Autodesk Inventor part; units mm, degrees
ref_plane "Work Plane1" through (0, 0, -6.2) normal (0, 0, -1) x (-1, 0, 0)
ref_plane "YZ Plane" through (0, 0, 0) normal (1, 0, 0) x (0, 1, 0)
ref_plane "XZ Plane" through (0, 0, 0) normal (0, 1, 0) x (-1, 0, 0)
sketch "Sketch1" plane through (0, 0, 0) normal (0, 0, 1) x (1, 0, 0)
  circle A0 centre (0, 0) radius 9.375
  dimension "d0" = 18.75
extrude "Extrusion1" add sketch "Sketch1" along normal blind 32
sketch "Sketch2" plane through (0, 0, 32) normal (0, 0, 1) x (1, 0, 0)
  circle A0 centre (0, 0) radius 9.375
  circle A1 centre (0, 0) radius 6.8
  dimension "d3" = 13.6
extrude "Extrusion2" add sketch "Sketch2" along normal blind 3.3 contours A1
sketch "Sketch3" plane through (0, 0, 32) normal (0, 0, 1) x (1, 0, 0)
  circle A0 centre (0, 0) radius 6.8
  line L0 (-3.25, 8) -> (3.25, 8)
  line L1 (-3.25, -8) -> (3.25, -8)
  line L2 (-3.25, 8) -> (-3.25, 6.8)
  line L3 (-3.25, 6.8) -> (3.25, 6.8)
  line L4 (3.25, 6.8) -> (3.25, 8)
  line L5 (-3.25, -8) -> (-3.25, -6.8)
  line L6 (-3.25, -6.8) -> (3.25, -6.8)
  line L7 (3.25, -6.8) -> (3.25, -8)
  dimension "d6" = 6.5
  dimension "d7" = 6.5
  dimension "d8" = 3.25
  dimension "d9" = 3.25
  dimension "d10" = 1.2
  dimension "d11" = 1.2
  dimension "d12" = 16
  dimension "d13" = 8
extrude "Extrusion3" add sketch "Sketch3" along normal blind 13 contours L6 L7 L1 L5 | L3 L2 L0 L4
sketch "Sketch4" plane through (-3.25, -8, 32) normal (0, -1, 0) x (1, 0, 0)
  line L0 (6.5, 0) -> (6.5, 13)
  line L1 (0, 13) -> (6.5, 13)
  circle A0 centre (3.25, 9.2) radius 1.7
  point P0 (3.25, -32)
  dimension "d16" = 3.4
  dimension "d17" = 3.25
  dimension "d18" = 3.8
extrude "Extrusion4" cut sketch "Sketch4" against normal up to surface (16 mm away)
fillet "Fillet1" radius 3.25 4 edges at (-3.25, -7.4, 45) (3.25, -7.4, 45) (-3.25, 7.4, 45) (3.25, 7.4, 45)
sketch "Sketch5" plane through (-3.25, 6.8, 32) normal (0, -1, 0) x (1, 0, 0)
  circle A0 centre (3.25, 9.2) radius 1.7
  circle A1 centre (3.25, 9.2) radius 1.95
  point P0 (3.25, -32)
  dimension "d22" = 3.9
extrude "Extrusion5" add sketch "Sketch5" along normal blind 1.2
sketch "Sketch6" plane through (0, -6.8, 32) normal (0, 1, 0) x (1, 0, 0)
  circle A0 centre (0, -9.2) radius 1.7
  circle A1 centre (0, -9.2) radius 1.95
  point P0 (0, 32)
  dimension "d25" = 3.9
extrude "Extrusion6" add sketch "Sketch6" along normal blind 1.2
sketch "Sketch7" plane through (0, 0, 0) normal (0, 0, -1) x (-1, 0, 0)
  circle A0 centre (0, 0) radius 9.375
  circle A1 centre (0, 0) radius 10.95
  dimension "d28" = 21.9
ref_plane "Work Plane1" through (0, 0, -6.2) normal (0, 0, -1) x (-1, 0, 0)
sketch "Sketch8" plane through (0, 0, -6.2) normal (0, 0, -1) x (-1, 0, 0)
  circle A0 centre (0, 0) radius 9.375
  circle A1 centre (0, 0) radius 8.75
  dimension "d30" = 17.5
loft "Loft1" add profiles "Sketch7", "Sketch8" contours A0 | A1 / A1
sketch "Sketch9" plane through (0, 0, 32) normal (0, 0, 1) x (1, 0, 0)
  circle A0 centre (0, 0) radius 9.375
  line L0 (-4.359, 8.3) -> (4.359, 8.3)
  line L1 (-4.359, -8.3) -> (4.359, -8.3)
  point P0 (8.3, 4.359)
  point P1 (8.3, -4.359)
  point P2 (-8.3, 4.359)
  point P3 (-8.3, -4.359)
  dimension "d51" = 16.6
  dimension "d52" = 8.3
thread "Thread1"
thread "Thread2"
thread "Thread3"
thread "Thread4"
sketch "Sketch10" plane through (0, 0, -6.2) normal (0, 0, -1) x (-1, 0, 0)
  circle A0 centre (0, 0) radius 8.75
  circle A1 centre (0, 0) radius 4.9
  circle A2 centre (0, 0) radius 3.8
  dimension "d47" = 9.8
  dimension "d48" = 7.6
extrude "Extrusion8" cut sketch "Sketch10" against normal blind 6 contours A1
extrude "Extrusion9" cut sketch "Sketch9" against normal up to surface (32 mm away) contours L0 A0 | A0 L1
sketch "Sketch11" plane through (0, 0, -6.2) normal (0, 0, -1) x (-1, 0, 0)
  circle A0 centre (0, 0) radius 3.8
  circle A1 centre (0, 0) radius 8.75
  circle A2 centre (0, 0) radius 4.9
  line L0 (6.1, 0.75) -> (1.7, 0.75)
  line L1 (1.7, 0.75) -> (1.7, -0.75)
  line L2 (1.7, -0.75) -> (6.1, -0.75)
  line L3 (6.1, -0.75) -> (6.1, 0.75)
  circle A3 centre (0, 0) radius 4.9
  line L4 (0.75, -4.8423) -> (0.75, -6.1)
  line L5 (0.75, -6.1) -> (-0.75, -6.1)
  line L6 (-0.75, -6.1) -> (-0.75, -4.8423)
  dimension "d55" = 4.4
  dimension "d56" = 1.5
  dimension "d57" = 1.5
  dimension "d58" = 1.2
  dimension "d59" = 0.75
  dimension "d60" = 1.2
  dimension "d61" = 0.75
extrude "Extrusion10" cut sketch "Sketch11" against normal up to surface (6 mm away) contours A0 L2 L1 L0 | A0 L0 A2 L2 | L0 L3 L2 A2 | A2 L4 L5 L6 picked at (2.4, 0) picked at (4.1442, -0.4181)
properties part number "KeySwitchBody" material "Steel, Alloy"
Check sheet for the modelled part. Datum: model origin and axes. Units: mm. A direction names the side the tool comes from. Round coordinates to 2 decimals unless told otherwise and drop trailing zeros. Order: outer loops, then holes, each group sorted by start corner. A loop starts at its lowest first (then second) coordinate and runs counter-clockwise, first axis right, second up. Notation, with made-up numbers: (81.25, 56.25) -> (128.25, 56.25) arc R25 ccw to (128.25, 70.25) -> close; hole circle Ø2 at (61.5, 38.25). An arc over 180 degrees is marked (long way). Use CSV: the item, a comma, the result in double quotes.
(1) Depth check by flat-ended pin: pin 1 (8.5 mm diameter, centred on x = -4, y = 4, fed in from +Z); pin 2 (10 mm diameter, centred on y = 5, z = 13, fed in from -X) (3 decimals); pin 3 (0.6 mm diameter, centred on x = -2.5, z = -2.5, fed in from +Y); pin 4 (3 mm diameter, centred on x = 0, z = 41.2, fed in from -Y). Enter the tip coordinate at first touch or a pass-through.
Worked out:
pin 1,"z = 44.9"
pin 2,"x = -9.375"
pin 3,"y = 9.88"
pin 4,"through"
(2) Material ranges on line 1 along Z through (x, y) = (0, -6.7); line 2 along Y through (x, z) = (2.5, 36.5); line 3 along X through (y, z) = (0, -2.65), recorded low to high. Write a range as from..to.
Worked out:
line 1,"-6.2..35.3, 39.25..39.5, 42.9..43.15"
line 2,"-8..-6.8, 6.8..8"
line 3,"-10.01..-6.1, -1.7..3.8, 4.9..10.01"
(3) Tool access check on faces 4 (the face through (-3.25, -7, 37)), 5 (the face through (-9.374, -0.143, 15.776)), 6 (the face through (-3.43, -3.5, -3.24)), 7 (the face through (0, 6.8, 37)). Record the directions out of +Z, -Z, +X, -X, +Y, -Y that give a thin tool (end or side, any length) a straight path to the whole face; none if there is none.
Worked out:
face 4,"+Z, -X, -Y"
face 5,"+Z, -X"
face 6,"-Z"
face 7,"none"
(4) Cross-section at B-B (y = 6.25). Count the separate pieces of the cut face and the enclosed holes in it, and give its area (3 significant figures).
Worked out:
separate pieces,"2"
enclosed holes,"1"
area,"562 mm²"
(5) Draft check along X on faces 1 (the face through (2.273, 7.408, 44.073)), 2 (the face through (0, -6.1, -3)), 3 (the face through (-2.323, -7.392, 44.023)). Enter one of: pulls with the +X half, pulls with the -X half, needs draft (parallel to the pull), parting line crosses it, or undercut.
Worked out:
face 1,"pulls with the +X half"
face 2,"undercut"
face 3,"pulls with the -X half"
(6) Cross-section at A-A (z = 41.2). Record the boundary of the cut face in (x, y).
Worked out:
outline,"(-3.25, -8) -> (-1.7, -8) -> (-1.7, -5.6) -> (-1.95, -5.6) -> (-1.95, -6.8) -> (-3.25, -6.8) -> close; (-3.25, 6.8) -> (-1.95, 6.8) -> (-1.95, 5.6) -> (-1.7, 5.6) -> (-1.7, 8) -> (-3.25, 8) -> close; (1.7, -8) -> (3.25, -8) -> (3.25, -6.8) -> (1.95, -6.8) -> (1.95, -5.6) -> (1.7, -5.6) -> close; (1.7, 5.6) -> (1.95, 5.6) -> (1.95, 6.8) -> (3.25, 6.8) -> (3.25, 8) -> (1.7, 8) -> close"
(7) Cross-section at C-C (z = 8). Record the boundary of the cut face in (x, y) (3 decimals).
Worked out:
outline,"(-4.359, -8.3) -> (4.359, -8.3) arc R9.375 ccw to (4.359, 8.3) -> (-4.359, 8.3) arc R9.375 ccw to start"
